Autodesk Fusion 360 part; units mm, degrees
sketch "Sketch1" plane through (0, 0, 0) normal (0, 0, 1) x (1, 0, 0)
  line L0 (0, 0) -> (18, 0) construction
  line L1 (18, 18) -> (18, 50)
  line L2 (0, 50) -> (0, 0)
  line L3 (0, 0) -> (50, 0)
  line L4 (50, 18) -> (18, 18)
  line L5 (0, 18) -> (0, 0) construction
  line L6 (53, 21) -> (21, 21)
  line L7 (21, 21) -> (21, 53)
  line L8 (-3, 53) -> (-3, -3)
  line L9 (-3, -3) -> (53, -3)
  line L10 (50, 18) -> (53, 18)
  line L11 (50, 0) -> (53, 0)
  line L12 (0, 50) -> (0, 53)
  line L13 (18, 50) -> (18, 53)
  line L14 (21, 53) -> (18, 53)
  line L15 (0, 53) -> (-3, 53)
  line L16 (53, -3) -> (53, 0)
  line L17 (53, 18) -> (53, 21)
  dimension "d1" = 18
  dimension "d2" = 50
  dimension "d3" = 50
  dimension "d4" = 18
extrude "Extrude1" add sketch "Sketch1" along normal blind 20 makes body 1 at (18, 29.6667, 13.3333) makes body 2 at (15.6667, -3, 6.6667)
sketch "Sketch2" plane through (0, 0, 0) normal (0, 0, -1) x (1, 0, 0)
  line L0 (53, -18) -> (18, -18)
  line L1 (18, -18) -> (18, -53)
  line L2 (18, -53) -> (21, -53)
  line L3 (21, -53) -> (21, -21)
  line L4 (21, -21) -> (53, -21)
  line L5 (53, -21) -> (53, -18)
  line L6 (0, -53) -> (0, 0)
  line L7 (0, 0) -> (53, 0)
  line L8 (53, 0) -> (53, 3)
  line L9 (53, 3) -> (-3, 3)
  line L10 (-3, 3) -> (-3, -53)
  line L11 (-3, -53) -> (0, -53)
  line L12 (-3, 3) -> (53, 3) construction
  line L13 (53, 3) -> (53, -21)
  line L14 (53, -21) -> (21, -53)
  line L15 (21, -53) -> (-3, -53)
  line L16 (-3, -53) -> (-3, 3)
  line L17 (-3, 3) -> (53, 3)
extrude "Extrude2" add sketch "Sketch2" along normal blind 2 bodies 1 2
fillet "Fillet1" radius 5 2 edges at (21, 21, 10) (-3, -3, 9) on bodies 1
fillet "Fillet2" radius 2 6 edges at (27.5, -3, -2) (-1.5355, -1.5355, -2) (-3, 27.5, -2) (39.5, 21, 0) (22.4645, 22.4645, 0) (21, 39.5, 0) on bodies 1
Build history of the part. All positions in model axes, mm. A direction names the side the tool comes from. Round coordinates to 2 decimals unless told otherwise and drop trailing zeros. Write each loop counter-clockwise with the first axis right and the second up, starting at its lowest first coordinate (ties: lowest second). Pieces come first, ordered by that corner, then holes. Notation, with made-up numbers: M 74,23 L 98,23 A25 ccw 98,47 Z; hole C 34.25,23.5 d4. An arc over 180 degrees is marked long. Answer as a JSON object with one key per item and string values. Group by question number.
(1) Flat gauge pins, fed straight in: pin 1 (5.5 mm diameter, centred on x = 43.5, z = 7.5, fed in from +Y); pin 2 (4 mm diameter, centred on y = 28.5, z = 4, fed in from +X); pin 3 (4 mm diameter, centred on x = 14, z = 8.5, fed in from +Y). Where does each tip first touch, or does it go through?
(2) Cut at A-A (z = 14.5). Give the cut face in (x, y).
(3) Mould opens along X. For faces 4 (the cylindrical face through (22, 23, 11)), 5 (the cylindrical face through (27.14, -2.4, -1.43)), 6 (the flat face through (18, 35, 10)), 7 (the flat face through (0, 27, 10)) say: pulls with the +X half, pulls with the -X half, needs draft (parallel to the pull), parting line crosses it, or undercut.
(4) Cut at D-D (x = 20). Give the cut face in (y, z).
(5) Drill centre lines: L1, parallel to X at y = 47.5, z = 2; L2, parallel to Y at x = 19.5, z = 15.5. Where is each one in solid material? Low to high.
(6) Cut at B-B (x = 12). Give the cut face in (y, z), and give its area (3 significant figures).
(7) Which spindle directions (+Z, -Z, +X, -X, +Y, -Y) get a long thin tool onto all of the face, cutting with end or side? Do faces 1 (the flat face through (40, 21, 11)), 2 (the flat face through (26, 0, 10)), 3 (the flat face through (20, 14, 0)). Say none if no direction does.
(8) Cut at C-C (y = 41.5). Give the cut face in (x, z), and give its area (3 significant figures).
Responses:
{
 "1": {"pin 1": "stops at y = 21", "pin 2": "stops at x = 21", "pin 3": "stops at y = 0"},
 "2": {"outline": "M -3,2 A5 ccw 2,-3 L 53,-3 L 53,0 L 0,0 L 0,53 L -3,53 Z; M 18,18 L 53,18 L 53,21 L 26,21 A5 cw 21,26 L 21,53 L 18,53 Z"},
 "3": {"face 4": "pulls with the +X half", "face 5": "needs draft", "face 6": "undercut", "face 7": "undercut"},
 "4": {"outline": "M -3,0 A2 ccw -1,-2 L 53,-2 L 53,20 L 18,20 L 18,0 L 0,0 L 0,20 L -3,20 Z"},
 "5": {"L1": "x = -3 to 0, 18 to 21", "L2": "y = -3 to 0, 18 to 53"},
 "6": {"outline": "M -3,0 A2 ccw -1,-2 L 53,-2 L 53,0 L 0,0 L 0,20 L -3,20 Z", "area": "171 mm2"},
 "7": {"face 1": "+Z, +X, +Y", "face 2": "+Z, +X", "face 3": "+Z"},
 "8": {"outline": "M -3,0 A2 ccw -1,-2 L 32.5,-2 L 32.5,0 L 23,0 A2 cw 21,2 L 21,20 L 18,20 L 18,0 L 0,0 L 0,20 L -3,20 Z", "area": "191 mm2"}
}
